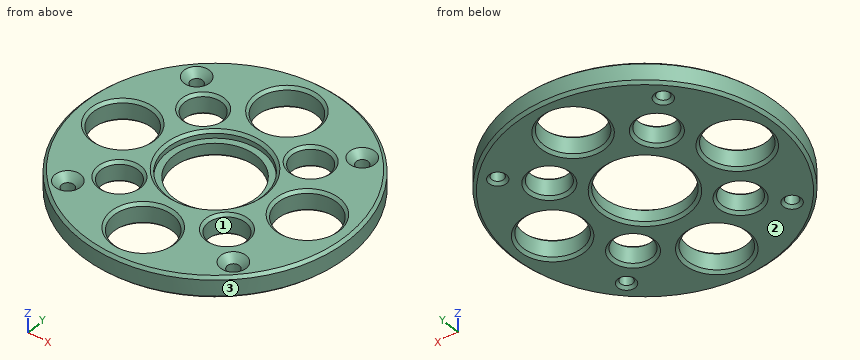
```python
from build123d import *

# Parameters (mm, degrees)
SKETCH006_R     = 50
SKETCH006_R_2   = 2.25
SKETCH006_R_3   = 15.5
SKETCH006_R_4   = 11
SKETCH006_R_5   = 7
PAD004_DEPTH    = 8
SKETCH007_R     = 17.85
POCKET002_DEPTH = 2.8
CHAMFER004_SIZE = 2.5
CHAMFER005_SIZE = 1


with BuildPart() as part:
    # Sketch006 → Pad004 (new body)
    with BuildSketch(Plane.XY):
        Circle(SKETCH006_R)
        with Locations((-30.479838, 30.479838)):
            Circle(SKETCH006_R_2, mode=Mode.SUBTRACT)
        with Locations((30.479838, 30.479838)):
            Circle(SKETCH006_R_2, mode=Mode.SUBTRACT)
        with Locations((30.479838, -30.479838)):
            Circle(SKETCH006_R_2, mode=Mode.SUBTRACT)
        with Locations((-30.479838, -30.479838)):
            Circle(SKETCH006_R_2, mode=Mode.SUBTRACT)
        Circle(SKETCH006_R_3, mode=Mode.SUBTRACT)
        with Locations((34, 0)):
            Circle(SKETCH006_R_4, mode=Mode.SUBTRACT)
        with Locations((0, -34)):
            Circle(SKETCH006_R_4, mode=Mode.SUBTRACT)
        with Locations((0, 34)):
            Circle(SKETCH006_R_4, mode=Mode.SUBTRACT)
        with Locations((-34, 0)):
            Circle(SKETCH006_R_4, mode=Mode.SUBTRACT)
        with Locations((-19.79899, 19.79899)):
            Circle(SKETCH006_R_5, mode=Mode.SUBTRACT)
        with Locations((19.79899, -19.79899)):
            Circle(SKETCH006_R_5, mode=Mode.SUBTRACT)
        with Locations((19.79899, 19.79899)):
            Circle(SKETCH006_R_5, mode=Mode.SUBTRACT)
        with Locations((-19.79899, -19.79899)):
            Circle(SKETCH006_R_5, mode=Mode.SUBTRACT)
    extrude(amount=PAD004_DEPTH)

    # Sketch007 → Pocket002 (cut)
    with BuildSketch(Plane.XY.offset(8)):
        Circle(SKETCH007_R)
    extrude(amount=-POCKET002_DEPTH, mode=Mode.SUBTRACT)

    # Chamfer004
    chamfer004_edges = [part.edges().sort_by_distance(p)[0] for p in [
        (28.229838, 30.479838, 8),
        (28.229838, -30.479838, 8),
        (-32.729838, -30.479838, 8),
        (-32.729838, 30.479838, 8),
    ]]
    chamfer(chamfer004_edges, length=CHAMFER004_SIZE)

    # Chamfer005
    chamfer005_edges = [part.edges().sort_by_distance(p)[0] for p in [
        (-50, 0, 8),
        (12.79899, 19.79899, 8),
        (23, 0, 8),
        (12.79899, -19.79899, 8),
        (-11, -34, 8),
        (-26.79899, -19.79899, 8),
        (-45, 0, 8),
        (-26.79899, 19.79899, 8),
        (-17.85, 0, 8),
        (-50, 0, 0),
        (-15.5, 0, 0),
        (-45, 0, 0),
        (-11, 34, 0),
        (-11, -34, 0),
        (23, 0, 0),
        (-26.79899, -19.79899, 0),
        (12.79899, 19.79899, 0),
        (12.79899, -19.79899, 0),
        (-26.79899, 19.79899, 0),
        (-32.729838, -30.479838, 0),
        (28.229838, -30.479838, 0),
        (28.229838, 30.479838, 0),
        (-32.729838, 30.479838, 0),
        (-11, 34, 8),
    ]]
    chamfer(chamfer005_edges, length=CHAMFER005_SIZE)


solid = part.part
```
For this review, take the finished solid that the model builds, in its own axes (mm). Face numbers are marked on the shaded views. Give positions to 0.01 mm unless a question says otherwise; leave off trailing zeros. One line per item, written item: value. Start each with the question number.
Q1. Draft analysis for pull direction X (two halves, no side actions). For the marked faces 1, 2 and 3, state which applies: released by +X, released by -X, zero draft, split by the parting line, or undercut.
Q2. Add section A-A (x = 0). Count the separate pieces of the cut face and the enclosed holes in it, and give its area (3 significant figures).
Q3. Clearance check with flat-ended pins moving along their axes: pin 1 Ø10.5 at (x, y) = (-5, -0.5) entering from +Z; pin 2 Ø7 at (x, y) = (-30.48, -30.48) entering from +Z; pin 3 Ø5 at (x, y) = (30.48, 30.48) entering from +Z; pin 4 Ø1.5 at (x, z) = (-17.5, 3.5) entering from -Y. State where each tip first meets the part, or that it passes through.
Q4. For L1, parallel to Y at x = 0, z = 2.6; L2, parallel to X at y = -4, z = 5.5; L3, parallel to X at y = 24, z = 6.75, list the stretches that pass through material, from the lowest coordinate up.
Reply:
1. face 1: undercut
1. face 2: zero draft
1. face 3: split by the parting line
2. separate pieces: 4
2. enclosed holes: 0
2. area: 179 mm²
3. pin 1: through
3. pin 2: z = 6.75
3. pin 3: z = 5.75
3. pin 4: y = -47.11
4. L1: -50 to -45, -23 to -15.5, 15.5 to 23, 45 to 50
4. L2: -49.84 to -44.25, -23.75 to -17.4, 17.4 to 23.75, 44.25 to 49.84
4. L3: -43.86 to -25.4, -14.2 to -4.58, 4.58 to 14.2, 25.4 to 43.86
